Here's how the part is built. I have some questions about the finished solid (model axes, mm). A direction names the side the tool comes from. Round coordinates to 2 decimals unless told otherwise and drop trailing zeros. Write each loop counter-clockwise with the first axis right and the second up, starting at its lowest first coordinate (ties: lowest second). Pieces come first, ordered by that corner, then holes. Notation, with made-up numbers: (23.25, 12.5) - (45.25, 12.5) arc R16 cw to (45.25, 18.5) - close; hole circle Ø1 at (55, -1). An arc over 180 degrees is marked (long way). Write item = value, one per line. Start each with the question number.
Item 1: For P1, Ø4, axis at y = 3.5, z = 5, coming from the +X side; P2, Ø5, axis at x = -4, y = -6, coming from the -Z side; P3, Ø5, axis at y = -6.5, z = 14, coming from the -X side; P4, Ø6, axis at x = 3.5, z = 7.5, coming from the +Y side, each with a flat end and sliding along its axis, tell me the tip position at first contact or that it passes through.
Item 2: If we section it at B-B (x = 2.25): Please give me the cut outline in (y, z).
Item 3: Which directions (+Z, -Z, +X, -X, +Y, -Y) give clear straight access to the entire face, cutting with the end or side of a thin tool? Please do faces 1 (the face through (-10, -5, 5)), 2 (the face through (0, -5, 15)), 3 (the face through (0, 0, -5)), 4 (the face through (5, 5, 0)).
Item 4: If we section it at C-C (z = 1.25): Please give me the cut outline in (x, y).
Item 5: If we section it at D-D (y = 4.75): Please give me the cut outline in (x, z), and give its area (3 significant figures).
Item 6: If we section it at A-A (y = -1.5): Please give me the cut outline in (x, z).
Item 7: If I drill on line 1 along Z through (x, y) = (-0.5, -5); line 2 along Y through (x, z) = (1.75, 18.25), over which ranges is the centre line in solid material (lowest first)? Write a range as [from, to].
```python
from build123d import *

# Parameters (mm, degrees)
F0_W     = 10
F0_H     = 10
F1_DEPTH = 20
F2_W     = 10
F2_H     = 10
F3_DEPTH = 10
F4_W     = 10
F4_H     = 10
F5_DEPTH = 10
F6_W     = 10
F6_H     = 10
F7_DEPTH = 10
F8_W     = 10
F8_H     = 10
F9_DEPTH = 10


with BuildPart() as f1:
    # F0 (on Top) → F1 (new body)
    with BuildSketch(Plane.XY):
        with Locations((5, -5)):
            Rectangle(F0_W, F0_H)
    extrude(amount=F1_DEPTH)

    # F2 (on Right) → F3 (join)
    with BuildSketch(Plane.YZ):
        with Locations((-5, 5)):
            Rectangle(F2_W, F2_H)
    extrude(amount=F3_DEPTH)

    # F4 (on Right) → F5 (join)
    with BuildSketch(Plane.YZ):
        with Locations((-5, 5)):
            Rectangle(F4_W, F4_H)
    extrude(amount=-F5_DEPTH)

    # F6 (on face) → F7 (join)
    with BuildSketch(Plane(origin=(0, 0, 0), x_dir=(1, 0, 0), z_dir=(0, 0, -1))):
        with Locations((5, 5)):
            Rectangle(F6_W, F6_H)
    extrude(amount=F7_DEPTH)

    # F8 (on Front) → F9 (join)
    with BuildSketch(Plane.XZ):
        with Locations((5, -5)):
            Rectangle(F8_W, F8_H)
    extrude(amount=-F9_DEPTH)


solid = f1.part
```
Reply:
q1.P1 = through
q1.P2 = 0
q1.P3 = 0
q1.P4 = 0
q2.outline = (-10, -10) - (10, -10) - (10, 0) - (0, 0) - (0, 20) - (-10, 20) - close
q3.face_1 = +Z, -Z, -X, +Y, -Y
q3.face_2 = +Z, -X, +Y, -Y
q3.face_3 = -Z, -X, +Y, -Y
q3.face_4 = +Z, +X, -X, +Y
q4.outline = (-10, -10) - (10, -10) - (10, 0) - (-10, 0) - close
q5.outline = (0, -10) - (10, -10) - (10, 0) - (0, 0) - close
q5.area = 100 mm2
q6.outline = (-10, 0) - (0, 0) - (0, -10) - (10, -10) - (10, 20) - (0, 20) - (0, 10) - (-10, 10) - close
q7.line_1 = [0, 10]
q7.line_2 = [-10, 0]
